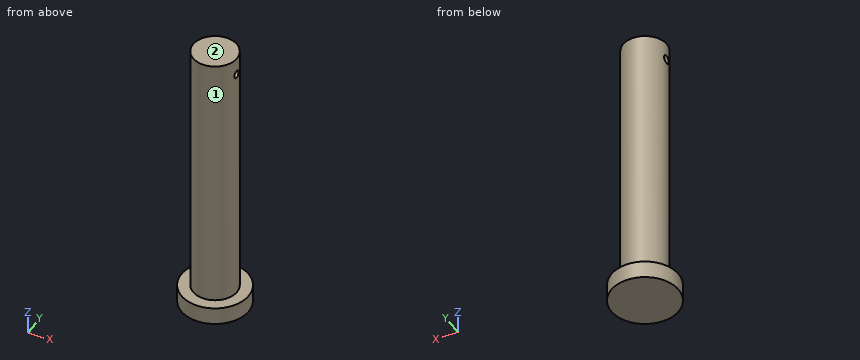
```python
from build123d import *

# Parameters (mm, degrees)
SKETCH2_R           = 23
BOSS_EXTRUDE1_DEPTH = 12
SKETCH3_R           = 15
BOSS_EXTRUDE2_DEPTH = 180
SCALE1_SCALE        = 0.3


with BuildPart() as part:
    # Sketch2 → Boss-Extrude1 (new body)
    with BuildSketch(Plane.XY):
        Circle(SKETCH2_R)
    extrude(amount=BOSS_EXTRUDE1_DEPTH)

    # Sketch3 → Boss-Extrude2 (add)
    with BuildSketch(Plane.XY.offset(12)):
        with Locations(Location((0, 0, 0), (0, 0, 180))):
            Circle(SKETCH3_R)
    extrude(amount=BOSS_EXTRUDE2_DEPTH)

    # Sketch4 → Cut-Revolve1 (revolve, cut)
    with BuildSketch(Plane.XY.offset(180), mode=Mode.PRIVATE) as cut_revolve1_sk:
        Polygon((-30, 0), (-30, 3), (30, 2.5), (30, 0), align=None)
    revolve(cut_revolve1_sk.sketch.rotate(Axis((30, 0, 180), (-1, 0, 0)), 137.024045149), axis=Axis((30, 0, 180), (-1, 0, 0)), mode=Mode.SUBTRACT)


with BuildPart() as part_1:
    # Scale1: scaled about (0.002156445, -4e-08, 88.550522263)
    add(part.part.scale(SCALE1_SCALE).moved(Location((0.001509511, -2.8e-08, 61.985365584))))


solid = part_1.part
```
The model under review builds one solid part; all positions refer to its coordinate system, in mm. Face numbers are marked on the shaded views. A direction names the side the tool comes from. Coordinates: 2 decimals unless noted, no trailing zeros. Write each loop counter-clockwise with the first axis right and the second up, starting at its lowest first coordinate (ties: lowest second). Pieces come first, ordered by that corner, then holes.
1) We need section C-C on z = 102. State the section outline as (x, y) points, then the cut area to 3 significant figures.
2) We need section D-D on y = 1.75. State the section outline as (x, z) points, then the cut area to 3 significant figures.
3) Machinability: for the marked faces 1 and 2, which of the approach directions +Z, -Z, +X, -X, +Y, -Y give a long, thin tool a straight path to every point of the face, cutting with its end or side? Answer none if there is none.
4) We need section B-B on y = -3.5. State the section outline as (x, z) points, then the cut area to 3 significant figures.
5) To check wall thickness, follow probe 1 along Z at (x, y) = (-3.25, -6); probe 2 along X at (y, z) = (-0.25, 72); probe 3 along X at (y, z) = (0.75, 102). State the ranges of each line that lie inside material, in increasing order.
6) Clearance check with flat-ended pins moving along their axes: pin 1 Ø1 at (x, z) = (2, 85.5) entering from +Y; pin 2 Ø2 at (y, z) = (-3, 84) entering from +X; pin 3 Ø3 at (y, z) = (1, 107) entering from -X. State where each tip first meets the part, or that it passes through.
7) We need section A-A on x = 1.75. State the section outline as (y, z) points.
Answer list:
1. outline: circle Ø9 at (0, 0)
1. area: 63.6 mm2
2. outline: (-6.67, 61.99) - (6.68, 61.99) - (6.68, 65.59) - (4.15, 65.59) - (4.15, 119.59) - (-4.14, 119.59) - (-4.14, 65.59) - (-6.67, 65.59) - close
2. area: 496 mm2
3. face 1: +Z
3. face 2: +Z, +X, -X, +Y, -Y
4. outline: (-5.94, 61.99) - (5.95, 61.99) - (5.95, 65.59) - (2.83, 65.59) - (2.83, 119.59) - (-2.83, 119.59) - (-2.83, 65.59) - (-5.94, 65.59) - close
4. area: 348 mm2
5. probe 1: z = 61.99 to 65.59
5. probe 2: x = -4.49 to 4.49
5. probe 3: x = -4.44 to 4.44
6. pin 1: stops at y = 4.24
6. pin 2: stops at x = 4.03
6. pin 3: stops at x = -4.5
7. outline: (-6.67, 61.99) - (6.67, 61.99) - (6.67, 65.59) - (4.15, 65.59) - (4.15, 119.59) - (-4.15, 119.59) - (-4.15, 65.59) - (-6.67, 65.59) - close; hole circle Ø1.62 at (0, 115.99)
